```python
from build123d import *

# Parameters (mm, degrees)
SKETCH2_W           = 220
SKETCH2_H           = 125
BOSS_EXTRUDE1_DEPTH = 3
SKETCH3_W           = 80
SKETCH3_H           = 6
SKETCH3_W_2         = 85
CUT_EXTRUDE1_DEPTH  = 3
SKETCH4_W           = 10.189923803
SKETCH4_H           = 53
CUT_EXTRUDE2_DEPTH  = 3
SKETCH6_W           = 15
SKETCH6_H           = 4
CUT_EXTRUDE3_DEPTH  = 10


with BuildPart() as part:
    # Sketch2 → Boss-Extrude1 (new body)
    with BuildSketch(Plane(origin=(0, 0, 0), x_dir=(0, 0, -1), z_dir=(1, 0, 0))):
        with Locations((-110, 62.5)):
            Rectangle(SKETCH2_W, SKETCH2_H)
    extrude(amount=BOSS_EXTRUDE1_DEPTH)

    # Sketch3 → Cut-Extrude1 (cut)
    with BuildSketch(Plane.ZY):
        with Locations((40, 122)):
            Rectangle(SKETCH3_W, SKETCH3_H)
        with Locations((40, 3)):
            Rectangle(SKETCH3_W, SKETCH3_H)
        with Locations((177.5, 122)):
            Rectangle(SKETCH3_W_2, SKETCH3_H)
        with Locations((177.5, 3)):
            Rectangle(SKETCH3_W_2, SKETCH3_H)
    extrude(amount=-CUT_EXTRUDE1_DEPTH, mode=Mode.SUBTRACT)

    # Sketch4 → Cut-Extrude2 (cut)
    with BuildSketch(Plane.ZY):
        with Locations((16.315088301, 62.5)):
            Rectangle(SKETCH4_W, SKETCH4_H)
        with Locations((36.815088301, 62.5)):
            Rectangle(SKETCH4_W, SKETCH4_H)
        with Locations((57.315088301, 62.5)):
            Rectangle(SKETCH4_W, SKETCH4_H)
        with Locations((77.815088301, 62.5)):
            Rectangle(SKETCH4_W, SKETCH4_H)
        with Locations((98.315088301, 62.5)):
            Rectangle(SKETCH4_W, SKETCH4_H)
        with Locations((118.815088301, 62.5)):
            Rectangle(SKETCH4_W, SKETCH4_H)
        with Locations((139.315088301, 62.5)):
            Rectangle(SKETCH4_W, SKETCH4_H)
        with Locations((159.815088301, 62.5)):
            Rectangle(SKETCH4_W, SKETCH4_H)
        with Locations((180.315088301, 62.5)):
            Rectangle(SKETCH4_W, SKETCH4_H)
        with Locations((200.815088301, 62.5)):
            Rectangle(SKETCH4_W, SKETCH4_H)
    extrude(amount=-CUT_EXTRUDE2_DEPTH, mode=Mode.SUBTRACT)

    # Sketch6 → Cut-Extrude3 (cut)
    with BuildSketch(Plane.ZY):
        with Locations((180, 111.5)):
            Rectangle(SKETCH6_W, SKETCH6_H)
        with Locations((180, 13.5)):
            Rectangle(SKETCH6_W, SKETCH6_H)
    extrude(amount=-CUT_EXTRUDE3_DEPTH, mode=Mode.SUBTRACT)


solid = part.part
```
CAD build for the part. Positions are in the model's coordinates, mm. Round coordinates to 2 decimals unless told otherwise and drop trailing zeros. Write each loop counter-clockwise with the first axis right and the second up, starting at its lowest first coordinate (ties: lowest second). Pieces come first, ordered by that corner, then holes. Notation, with made-up numbers: (9.5, 1.5) - (22.5, 1.5) arc R12 ccw to (22.5, 7.5) - close; hole circle Ø6 at (36, 88.25). An arc over 180 degrees is marked (long way). Return JSON: item names as keys, results as strings. Group by question number.
Item 1: Band-saw the part on A-A on z = 56.5. List the corners of the cut face in (x, y), plus the area to 3 significant figures.
Item 2: Mould opens along X. For faces 1 (the face through (3, 63, 112)), 2 (the face through (0, 63, 112)) say: +X half, -X half, draft (parallel to the pull), parting line (faces both ways), or undercut.
Item 3: Probe probe 1 along Y at (x, z) = (2, 184.5); probe 2 along Y at (x, z) = (1.1, 101.5); probe 3 along Y at (x, z) = (1, 35). List the from-to ranges inside material, lowest first.
Item 4: Band-saw the part on C-C on x = 2.45. State how many separate pieces and enclosed holes the cut face has, plus the area to 3 significant figures.
Item 5: Flat gauge pins, fed straight in: pin 1 Ø0.9 at (x, y) = (1.5, 123) entering from -Z; pin 2 Ø1.5 at (x, z) = (1, 180.5) entering from +Y; pin 3 Ø1.5 at (x, z) = (2, 39.5) entering from -Y. Where does each tip first touch, or does it go through?
Item 6: Band-saw the part on B-B on z = 97.5. List the corners of the cut face in (x, y).
Resolved:
{
 "1": {"outline": "(0, 6) - (3, 6) - (3, 36) - (0, 36) - close; (0, 89) - (3, 89) - (3, 119) - (0, 119) - close", "area": "180 mm²"},
 "2": {"face 1": "+X half", "face 2": "-X half"},
 "3": {"probe 1": "y = 6 to 11.5, 15.5 to 36, 89 to 109.5, 113.5 to 119", "probe 2": "y = 0 to 36, 89 to 125", "probe 3": "y = 6 to 36, 89 to 119"},
 "4": {"separate pieces": "1", "enclosed holes": "12", "area": "20,000 mm²"},
 "5": {"pin 1": "stops at z = 80", "pin 2": "stops at y = 119", "pin 3": "stops at y = 6"},
 "6": {"outline": "(0, 0) - (3, 0) - (3, 36) - (0, 36) - close; (0, 89) - (3, 89) - (3, 125) - (0, 125) - close"}
}
